from build123d import *

# Parameters (mm, degrees)
BOSS_EXTRUDE1_DEPTH = 20
BOSS_EXTRUDE2_DEPTH = 17.5
SKETCH3_R           = 3.75
CUT_EXTRUDE1_DEPTH  = 21


with BuildPart() as part:
    # Sketch1 → Boss-Extrude1 (new body)
    with BuildSketch(Plane(origin=(0, 0, 0), x_dir=(0, 0, -1), z_dir=(1, 0, 0))):
        with BuildLine():
            Line((-8.75, 0), (8.75, 0))
            Line((8.75, 0), (8.75, 8.75))
            ThreePointArc((8.75, 8.75), (0, 17.5), (-8.75, 8.75))
            Line((-8.75, 8.75), (-8.75, 0))
        make_face()
    extrude(amount=BOSS_EXTRUDE1_DEPTH)

    # Sketch2 → Boss-Extrude2 (add)
    with BuildSketch(Plane.XZ):
        with BuildLine():
            Line((0, 12.75), (0, 8.75))
            Line((0, 8.75), (0, 0))
            Line((0, 0), (20, 0))
            Line((20, 0), (20, 8.75))
            Line((20, 8.75), (9, 8.75))
            ThreePointArc((9, 8.75), (5, 12.75), (9, 16.75))
            Line((9, 16.75), (17, 16.75))
            Line((17, 16.75), (17, 21.75))
            Line((17, 21.75), (9, 21.75))
            ThreePointArc((9, 21.75), (2.636038969, 19.113961031), (0, 12.75))
        make_face()
    extrude(amount=-BOSS_EXTRUDE2_DEPTH)

    # Sketch3 → Cut-Extrude1 (cut, through all)
    with BuildSketch(Plane.ZY):
        with Locations((0, 8.75)):
            Circle(SKETCH3_R)
    extrude(amount=-CUT_EXTRUDE1_DEPTH, mode=Mode.SUBTRACT)


solid = part.part
Work out the finished part from the listing and answer in its coordinate system (mm). A direction names the side the tool comes from. Round coordinates to 2 decimals unless told otherwise and drop trailing zeros. Order: outer loops, then holes, each group sorted by start corner. A loop starts at its lowest first (then second) coordinate and runs counter-clockwise, first axis right, second up. Notation, with made-up numbers: M 0.5,72 L 32.5,72 A9 cw 32.5,76 Z; hole C 55.5,88 d8. An arc over 180 degrees is marked long. Put each result on its own line as item: value. Start each with the question number.
Q1. Section A-A, the plane x = 14.75 is taken. Write down the section's boundary in (y, z), and give its area (3 significant figures).
Q2. Flat-ended cylindrical pins translate along their axes: pin 1 (1.5 mm diameter, centred on y = 10, z = 18, fed in from +X); pin 2 (5 mm diameter, centred on x = 4.5, y = 6, fed in from +Z). Find the tip coordinate at first contact, or state that the pin passes through.
Q3. Section D-D, the plane z = 19 is taken. Write down the section's boundary in (x, y), and give its area (3 significant figures).
Q4. Straight lines are drawn through the part: L1, parallel to Z at x = 16, y = 1.75; L2, parallel to Z at x = 13.75, y = 8.25; L3, parallel to Z at x = 15.75, y = 9.5. For each, find the intervals that lie inside material, in ascending order. Write a range as [from, to].
Q5. A tool of negligible diameter and unlimited length cuts with its end or side. For faces 5 (the flat face through (13, 9, 16.75)), 6 (the flat face through (0, 9, 5)), 7 (the flat face through (17, 9, 19)), from which of +Z, -Z, +X, -X, +Y, -Y can it reach the whole face along a straight path? Write none if from no direction.
Q6. Section C-C, the plane x = 18.75 is taken. Write down the section's boundary in (y, z).
Q7. Section B-B, the plane y = 11.25 is taken. Write down the section's boundary in (x, z), and give its area (3 significant figures).
Q8. For a pull along Z with two mould halves and no side action, classify faces 1 (the flat face through (10, 4, -8.75)), 2 (the cylindrical face through (9.86, 12.468, -0.488)), 3 (the flat face through (10, 0, 3)), 4 (the flat face through (13, 9, 21.75)) as pulls with the +Z half, pulls with the -Z half, needs draft (parallel to the pull), parting line crosses it, or undercut.
Findings below:
1. outline: M 0,-8.75 L 8.75,-8.75 A8.75 ccw 17.5,0 L 17.5,8.75 L 0,8.75 Z; M 0,16.75 L 17.5,16.75 L 17.5,21.75 L 0,21.75 Z; hole C 8.75,0 d7.5
1. area: 333 mm^2
2. pin 1: stops at x = 17
2. pin 2: stops at z = 21.52
3. outline: M 2.52,0 L 17,0 L 17,17.5 L 2.52,17.5 Z
3. area: 253 mm^2
4. L1: z = [-8.75, 8.75], [16.75, 21.75]
4. L2: z = [-8.75, -3.72], [3.72, 8.75], [16.75, 21.75]
4. L3: z = [-8.72, -3.67], [3.67, 8.75], [16.75, 21.75]
5. face 5: +X, +Y, -Y
5. face 6: +Z, -Z, -X, +Y, -Y
5. face 7: +Z, +X, +Y, -Y
6. outline: M 0,-8.75 L 8.75,-8.75 A8.75 ccw 17.5,0 L 17.5,8.75 L 0,8.75 Z; hole C 8.75,0 d7.5
7. outline: M 0,-8.39 L 20,-8.39 L 20,-2.8 L 0,-2.8 Z; M 0,2.8 L 20,2.8 L 20,8.75 L 9,8.75 A4 cw 9,16.75 L 17,16.75 L 17,21.75 L 9,21.75 A9 ccw 0,12.75 Z
7. area: 345 mm^2
8. face 1: pulls with the -Z half
8. face 2: undercut
8. face 3: needs draft
8. face 4: pulls with the +Z half
